The listing builds one solid part. Answer for the finished solid, in the listing's coordinates (mm). Give positions to 0.01 mm unless a question says otherwise; leave off trailing zeros. Loops run counter-clockwise (first coordinate to the right, second up) from the corner with the lowest first, then second, coordinate; pieces in that order, holes last. Notation, with made-up numbers: (66, 70.5) - (116, 70.5) arc R20 ccw to (116, 79.5) - close; hole circle Ø8 at (83.5, -26.75). An arc over 180 degrees is marked (long way). Answer as CSV lines item,"result". Start each with the question number.
1) A cutting plane is placed at C-C (x = -1). Determine the outline of the cut face in (y, z).
2) A cutting plane is placed at B-B (y = 209.5). Determine the outline of the cut face in (x, z) (3 decimals), and give its area (3 significant figures).
3) Find the intervals of material crossed by line 1 along Z through (x, y) = (-249, 98); line 2 along X through (y, z) = (-60.5, 26); line 3 along Y through (x, z) = (17.5, 43), in increasing order.
4) A cutting plane is placed at A-A (x = -176.5). Determine the outline of the cut face in (y, z).
5) Flat-ended cylindrical pins translate along their axes: pin 1 (12 mm diameter, centred on x = 171, y = 101, fed in from +Z); pin 2 (5 mm diameter, centred on x = 116.5, z = 43, fed in from -Y); pin 3 (2.5 mm diameter, centred on x = 287.5, y = -50.5, fed in from -Z); pin 4 (10 mm diameter, centred on x = -116.5, y = -99.5, fed in from -Z). Find the tip coordinate at first contact, or state that the pin passes through.
```python
from build123d import *

# Parameters (mm, degrees)
F0_W     = 571.5
F0_H     = 596.9
F1_DEPTH = 36.576
F2_W     = 577.85
F2_H     = 596.9
F3_DEPTH = 3.175
F4_W     = 508
F4_H     = 25.4
F4_W_2   = 76.2
F5_DEPTH = 6.35


with BuildPart() as f1:
    # F0 (on Top) → F1 (new body)
    with BuildSketch(Plane.XY):
        Rectangle(F0_W, F0_H)
    extrude(amount=F1_DEPTH)

    # F2 (on face) → F3 (join)
    with BuildSketch(Plane.XY.offset(36.576)):
        Rectangle(F2_W, F2_H)
    extrude(amount=F3_DEPTH)

    # F4 (on face) → F5 (join)
    with BuildSketch(Plane.XY.offset(39.751)):
        with Locations((0, -234.95)):
            Rectangle(F4_W, F4_H)
        with Locations((0, 247.65)):
            Rectangle(F4_W_2, F4_H)
    extrude(amount=F5_DEPTH)


solid = f1.part
```
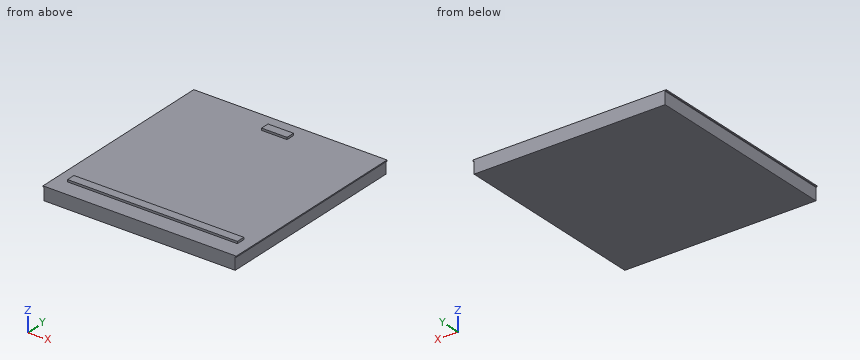
Ans:
1,outline,"(-298.45, 0) - (298.45, 0) - (298.45, 39.75) - (260.35, 39.75) - (260.35, 46.1) - (234.95, 46.1) - (234.95, 39.75) - (-222.25, 39.75) - (-222.25, 46.1) - (-247.65, 46.1) - (-247.65, 39.75) - (-298.45, 39.75) - close"
2,outline,"(-288.925, 36.576) - (-285.75, 36.576) - (-285.75, 0) - (285.75, 0) - (285.75, 36.576) - (288.925, 36.576) - (288.925, 39.751) - (-288.925, 39.751) - close"
2,area,"22,700 mm2"
3,line 1,"0 to 39.75"
3,line 2,"-285.75 to 285.75"
3,line 3,"-247.65 to -222.25, 234.95 to 260.35"
4,outline,"(-298.45, 0) - (298.45, 0) - (298.45, 39.75) - (-222.25, 39.75) - (-222.25, 46.1) - (-247.65, 46.1) - (-247.65, 39.75) - (-298.45, 39.75) - close"
5,pin 1,"z = 39.75"
5,pin 2,"y = -247.65"
5,pin 3,"z = 36.58"
5,pin 4,"z = 0"
